Geometry: final body of the model. Coordinates: model frame, mm. Face numbers are marked on the shaded views. A direction names the side the tool comes from. Give positions to 0.01 mm unless a question says otherwise; leave off trailing zeros. Loops run counter-clockwise (first coordinate to the right, second up) from the corner with the lowest first, then second, coordinate; pieces in that order, holes last.
from build123d import *

# Parameters (mm, degrees)
SALIENTE_EXTRUIR1_DEPTH = 2
SALIENTE_EXTRUIR2_DEPTH = 4
CORTAR_EXTRUIR1_REACH   = 19.066
CROQUIS3_R              = 1.5
CROQUIS4_W              = 1
CROQUIS4_H              = 6
SALIENTE_EXTRUIR3_DEPTH = 15


with BuildPart() as part:
    # Croquis1 → Saliente-Extruir1 (new body)
    with BuildSketch(Plane(origin=(0, 0, 0), x_dir=(1, 0, 0), z_dir=(0, 1, 0))):
        with BuildLine():
            Line((-9.5, 5.5), (9.5, 5.5))
            ThreePointArc((9.5, 5.5), (15, 0), (9.5, -5.5))
            Line((9.5, -5.5), (-9.5, -5.5))
            ThreePointArc((-9.5, -5.5), (-15, 0), (-9.5, 5.5))
        make_face()
    extrude(amount=SALIENTE_EXTRUIR1_DEPTH)

    # Croquis2 → Saliente-Extruir2 (add)
    with BuildSketch(Plane(origin=(0, 2, 0), x_dir=(1, 0, 0), z_dir=(0, 1, 0))):
        with BuildLine():
            Line((-3.2, 4), (-3.2, -4))
            Line((-3.2, -4), (-11.75, -4))
            Line((-11.75, -4), (-11.75, -4.1))
            ThreePointArc((-11.75, -4.1), (-11.486396103, -4.736396103), (-10.85, -5))
            Line((-10.85, -5), (10.85, -5))
            ThreePointArc((10.85, -5), (11.486396103, -4.736396103), (11.75, -4.1))
            Line((11.75, -4.1), (11.75, -4))
            Line((11.75, -4), (3.2, -4))
            Line((3.2, -4), (3.2, 4))
            Line((3.2, 4), (11.75, 4))
            Line((11.75, 4), (11.75, 4.1))
            ThreePointArc((11.75, 4.1), (11.486396103, 4.736396103), (10.85, 5))
            Line((10.85, 5), (-10.85, 5))
            ThreePointArc((-10.85, 5), (-11.486396103, 4.736396103), (-11.75, 4.1))
            Line((-11.75, 4.1), (-11.75, 4))
            Line((-11.75, 4), (-3.2, 4))
        make_face()
    extrude(amount=SALIENTE_EXTRUIR2_DEPTH)

    # Croquis3 → Cortar-Extruir1 (cut, up to next)
    with BuildSketch(Plane(origin=(0, 6, 0), x_dir=(1, 0, 0), z_dir=(0, 1, 0)), mode=Mode.PRIVATE) as cortar_extruir1_sk1:
        with Locations(Location((0, 0, 0), (0, 0, 270))):
            Circle(CROQUIS3_R)
    cortar_extruir1_tool1 = extrude(cortar_extruir1_sk1.sketch, amount=-CORTAR_EXTRUIR1_REACH, mode=Mode.PRIVATE) & part.part
    add(cortar_extruir1_tool1.solids().sort_by_distance((0, 6, 0))[0], mode=Mode.SUBTRACT)

    # Croquis4 → Saliente-Extruir3 (add)
    with BuildSketch(Plane.XZ):
        with Locations((-6.5, 0)):
            Rectangle(CROQUIS4_W, CROQUIS4_H)
        with Locations((6.5, 0)):
            Rectangle(CROQUIS4_W, CROQUIS4_H)
    extrude(amount=SALIENTE_EXTRUIR3_DEPTH)


solid = part.part
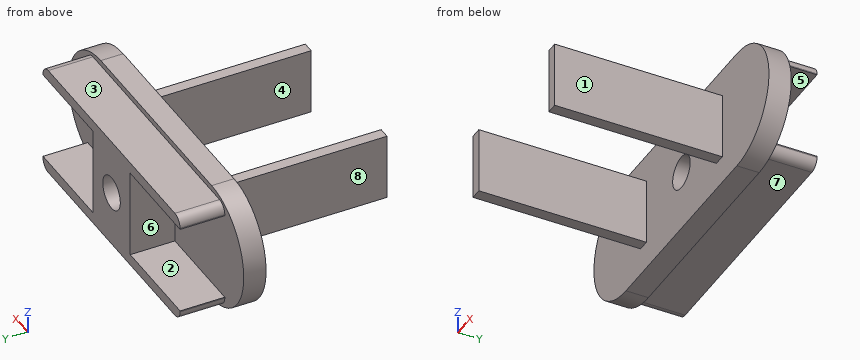
Item 1: Section query B-B on z = 0. Return loops of the section in (x, y).
Values follow:
outline: (-15, 0) - (-7, 0) - (-7, -15) - (-6, -15) - (-6, 0) - (-1.5, 0) - (-1.5, 6) - (-3.2, 6) - (-3.2, 2) - (-15, 2) - close; (1.5, 0) - (6, 0) - (6, -15) - (7, -15) - (7, 0) - (15, 0) - (15, 2) - (3.2, 2) - (3.2, 6) - (1.5, 6) - close
Item 2: Ray query, probe 1 along X at (y, z) = (-6.5, 2); probe 2 along X at (y, z) = (3.85, 0); probe 3 along Y at (x, z) = (-0.25, -3.75). Return the intervals inside material, ascending.
Values follow:
probe 1: x = -7 to -6, 6 to 7
probe 2: x = -3.2 to -1.5, 1.5 to 3.2
probe 3: y = 0 to 6
Item 3: Section query C-C on y = -4. Return loops of the section in (x, z).
Values follow:
outline: (-7, -3) - (-6, -3) - (-6, 3) - (-7, 3) - close; (6, -3) - (7, -3) - (7, 3) - (6, 3) - close
Item 4: Section query A-A on x = 0. Return loops of the section in (y, z).
Values follow:
outline: (0, -5.5) - (2, -5.5) - (2, -5) - (6, -5) - (6, -1.5) - (0, -1.5) - close; (0, 1.5) - (6, 1.5) - (6, 5) - (2, 5) - (2, 5.5) - (0, 5.5) - close
Item 5: Set-up query: the marked faces 4, 5, 6, 7 and 8. Return all of +Z, -Z, +X, -X, +Y, -Y with unobstructed straight access to the full face (end or side cutting, diameter ignored); none if empty.
Values follow:
face 4: +Z, -Z, -Y
face 5: +X, +Y
face 6: -X, +Y
face 7: -Z, +X, -X, +Y
face 8: +Z, -Z, -X, -Y
Item 6: Draft query along Z for the marked faces 1, 2 and 3. Return one class per face: +Z half, -Z half, draft (parallel to the pull), parting line (faces both ways), or undercut.
Values follow:
face 1: draft
face 2: undercut
face 3: +Z half
Item 7: Pin query (flat end, axial travel): pin 1 (5 mm diameter, centred on x = 2.5, z = 3.5, fed in from -Y); pin 2 (1 mm diameter, centred on x = -6.5, y = -1, fed in from +Z); pin 3 (2 mm diameter, centred on x = -4, y = 4, fed in from -Z). Return the tip coordinate at first contact, or that it passes through.
Values follow:
pin 1: stops at y = 0
pin 2: stops at z = 3
pin 3: stops at z = -5
Item 8: Section query D-D on y = 1.25. Return loops of the section in (x, z).
Values follow:
outline: (-9.5, -5.5) - (9.5, -5.5) arc R5.5 ccw to (9.5, 5.5) - (-9.5, 5.5) arc R5.5 ccw to start; hole circle Ø3 at (0, 0)
